```python
from build123d import *

# Parameters (mm, degrees)
SKETCH1_W           = 40
SKETCH1_H           = 40
BOSS_EXTRUDE1_DEPTH = 40
CUT_EXTRUDE1_DEPTH  = 40
SKETCH3_W           = 5
SKETCH3_H           = 20
CUT_EXTRUDE3_DEPTH  = 40
CUT_EXTRUDE4_DEPTH  = 40
SKETCH5_W           = 20
SKETCH5_H           = 20
CUT_EXTRUDE6_DEPTH  = 20
CUT_EXTRUDE8_DEPTH  = 20
BOSS_EXTRUDE3_DEPTH = 20


with BuildPart() as part:
    # Sketch1 → Boss-Extrude1 (new body)
    with BuildSketch(Plane.XY):
        with Locations((20, 20)):
            Rectangle(SKETCH1_W, SKETCH1_H)
    extrude(amount=BOSS_EXTRUDE1_DEPTH)

    # Sketch2 → Cut-Extrude1 (cut)
    with BuildSketch(Plane.XY.offset(40)):
        with BuildLine():
            ThreePointArc((0, 20), (5.857864376, 34.142135624), (20, 40))
            Line((20, 40), (0, 40))
            Line((0, 40), (0, 20))
        make_face()
        with BuildLine():
            ThreePointArc((20, 0), (5.857864376, 5.857864376), (0, 20))
            Line((0, 20), (0, 0))
            Line((0, 0), (20, 0))
        make_face()
    extrude(amount=-CUT_EXTRUDE1_DEPTH, mode=Mode.SUBTRACT)

    # Sketch3 → Cut-Extrude3 (cut)
    with BuildSketch(Plane(origin=(0, 40, 0), x_dir=(1, 0, 0), z_dir=(0, 1, 0))):
        with Locations((2.5, -30)):
            Rectangle(SKETCH3_W, SKETCH3_H)
    extrude(amount=-CUT_EXTRUDE3_DEPTH, mode=Mode.SUBTRACT)

    # Sketch4 → Cut-Extrude4 (cut)
    with BuildSketch(Plane(origin=(0, 0, 0), x_dir=(0, 0, -1), z_dir=(1, 0, 0))):
        Polygon((-20, 40), (-40, 20), (-40, 40), align=None)
    extrude(amount=CUT_EXTRUDE4_DEPTH, mode=Mode.SUBTRACT)

    # Sketch5 → Cut-Extrude6 (cut)
    with BuildSketch(Plane.XY.offset(40)):
        with Locations((30, 30)):
            Rectangle(SKETCH5_W, SKETCH5_H)
    extrude(amount=-CUT_EXTRUDE6_DEPTH, mode=Mode.SUBTRACT)

    # Sketch6 → Cut-Extrude8 (cut)
    with BuildSketch(Plane.XY.offset(40)):
        with BuildLine():
            Line((6.771243445, 5), (20, 20))
            Line((20, 20), (5, 20))
            Line((5, 20), (5, 6.771243445))
            ThreePointArc((5, 6.771243445), (5.857864376, 5.857864376), (6.771243445, 5))
        make_face()
        with BuildLine():
            Line((5, 20), (20, 20))
            Line((20, 20), (20, 40))
            ThreePointArc((20, 40), (1.771243445, 28.228756555), (5, 6.771243445))
            Line((5, 6.771243445), (5, 20))
        make_face()
    extrude(amount=-CUT_EXTRUDE8_DEPTH, mode=Mode.SUBTRACT)

    # Sketch7 → Boss-Extrude3 (add)
    with BuildSketch(Plane(origin=(40, 0, 0), x_dir=(0, 0, -1), z_dir=(1, 0, 0))):
        Polygon((-20, 40), (-40, 20), (-20, 20), align=None)
    extrude(amount=-BOSS_EXTRUDE3_DEPTH)


solid = part.part
```
Check sheet for the modelled part. Datum: model origin and axes. Units: mm. A direction names the side the tool comes from. Round coordinates to 2 decimals unless told otherwise and drop trailing zeros. Write each loop counter-clockwise with the first axis right and the second up, starting at its lowest first coordinate (ties: lowest second). Pieces come first, ordered by that corner, then holes. Notation, with made-up numbers: (-12, 86) -> (-1, 86) arc R31 ccw to (-1, 115) -> close; hole circle Ø10 at (71.25, -20). An arc over 180 degrees is marked (long way). One line per question, with ' | ' between items. Start each with the question number.
1. Sectioned sample at A-A, the plane z = 32. Record the cut outline in (x, y).
2. Depth check by flat-ended pin: pin 1 (10 mm diameter, centred on y = 12, z = 20.5, fed in from -X); pin 2 (1 mm diameter, centred on y = 31.5, z = 9.5, fed in from -X); pin 3 (1.5 mm diameter, centred on x = 5, z = 28.5, fed in from +Y); pin 4 (5 mm diameter, centred on x = 13.5, z = 9.5, fed in from +Y). Enter the tip coordinate at first touch or a pass-through.
3. Set-up check for faces 1 (the face through (27, 10, 40)), 2 (the face through (13.3, 12.4, 30.1)): record each of +Z, -Z, +X, -X, +Y, -Y from which the full face is reachable in a straight line by a thin tool's end or side.
4. Sectioned sample at B-B, the plane x = 26. Record the cut outline in (y, z), then the cut area to 3 significant figures.
5. Scan lines: line 1 along Z through (x, y) = (15.5, 28); line 2 along X through (y, z) = (29, 26); line 3 along X through (y, z) = (5, 11.5). Record each from-to range of solid material in increasing order. Write a range as from..to.
6. Sectioned sample at D-D, the plane z = 5.5. Record the cut outline in (x, y), then the cut area to 3 significant figures.
7. Sectioned sample at C-C, the plane y = 29.5. Record the cut outline in (x, z).
Taken from the geometry:
1) outline: (6.77, 5) arc R20 ccw to (20, 0) -> (40, 0) -> (40, 28) -> (20, 28) -> (20, 20) -> close
2) pin 1: stops at x = 0.23 | pin 2: stops at x = 3.3 | pin 3: passes through | pin 4: stops at y = 39.6
3) face 1: +Z, +X, -X, +Y, -Y | face 2: +Z, -X, +Y
4) outline: (0, 0) -> (40, 0) -> (40, 20) -> (20, 40) -> (0, 40) -> close | area: 1,400 mm^2
5) line 1: z = 0..20 | line 2: x = 20..40 | line 3: x = 6.77..40
6) outline: (20, 0) -> (40, 0) -> (40, 40) -> (20, 40) arc R20 ccw to start | area: 1,430 mm^2
7) outline: (2.4, 0) -> (40, 0) -> (40, 30.5) -> (20, 30.5) -> (20, 20) -> (2.4, 20) -> close
